from build123d import *

# Parameters (mm, degrees)
BLANKSKE_W         = 300
BLANKSKE_H         = 45
BLANK_DEPTH        = 30
TOOTHCUTSIM_DEPTH  = 305.836021494
TEETHCUTS_COUNT    = 20
TEETHCUTS_PITCH    = 15.70796325
SKETCH1_W          = 305.531648247
SKETCH1_H          = 78.813182986
CUT_EXTRUDE1_DEPTH = 15
SKETCH2_W          = 303.838018684
SKETCH2_H          = 48.852788509
CUT_EXTRUDE2_DEPTH = 26
SKETCH3_W          = 15
SKETCH3_H          = 19
CUT_EXTRUDE3_DEPTH = 138


with BuildPart() as part:
    # BlankSke → Blank (new body)
    with BuildSketch(Plane.XY):
        with Locations((150, 22.5)):
            Rectangle(BLANKSKE_W, BLANKSKE_H)
    extrude(amount=-BLANK_DEPTH)

    # TooCutSkeSim → ToothCutSim (cut, through all)
    with BuildSketch(Plane.XY):
        Polygon((2.153176848, 33.75), (-2.153176848, 33.75), (-6.257086828, 45.0254), (6.257086828, 45.0254), align=None)
    toothcutsim = extrude(amount=-TOOTHCUTSIM_DEPTH, mode=Mode.SUBTRACT)

    # TeethCuts: ToothCutSim ×20
    with Locations(*[(i * TEETHCUTS_PITCH, 0, 0) for i in range(1, TEETHCUTS_COUNT)]):
        add(toothcutsim, mode=Mode.SUBTRACT)

    # Sketch1 → Cut-Extrude1 (cut)
    with BuildSketch(Plane.XY):
        with Locations((152.765824124, 39.406591493)):
            Rectangle(SKETCH1_W, SKETCH1_H)
    extrude(amount=-CUT_EXTRUDE1_DEPTH, mode=Mode.SUBTRACT)

    # Sketch2 → Cut-Extrude2 (cut)
    with BuildSketch(Plane.XZ):
        with Locations((151.919009342, -5.573605746)):
            Rectangle(SKETCH2_W, SKETCH2_H)
    extrude(amount=-CUT_EXTRUDE2_DEPTH, mode=Mode.SUBTRACT)

    # Sketch3 → Cut-Extrude3 (cut)
    with BuildSketch(Plane(origin=(300, 0, 0), x_dir=(0, 0, -1), z_dir=(1, 0, 0))):
        with Locations((22.5, 35.5)):
            Rectangle(SKETCH3_W, SKETCH3_H)
    extrude(amount=-CUT_EXTRUDE3_DEPTH, mode=Mode.SUBTRACT)


solid = part.part
Geometry check sheet. Reference: the model listing, model coordinates, mm. A direction names the side the tool comes from. Coordinates: 2 decimals unless noted, no trailing zeros. Order: outer loops, then holes, each group sorted by start corner. A loop starts at its lowest first (then second) coordinate and runs counter-clockwise, first axis right, second up. Notation, with made-up numbers: (-20, 80.25) - (6, 80.25) arc R28 ccw to (6, 102.25) - close; hole circle Ø1 at (-16, 48.5). An arc over 180 degrees is marked (long way). One line per item, written item: value.
(1) Sectioned sample at C-C (x = 90.5). Enter the section's corners in (y, z).
Data:
outline: (26, -30) - (38.13, -30) - (38.13, -15) - (26, -15) - close
(2) Depth check by flat-ended pin: pin 1 Ø1.1 at (x, z) = (1.5, -19.5) entering from +Y. Enter the tip coordinate at first touch or a pass-through.
Data:
pin 1: stops at y = 33.75
(3) Sectioned sample at B-B (x = 129.5). Enter the section's corners in (y, z).
Data:
outline: (26, -30) - (38.37, -30) - (38.37, -15) - (26, -15) - close
(4) Access from +Z, -Z, +X, -X, +Y, -Y to the whole of each face (thin tool, end or side, straight path). Record for faces 1 (the face through (160.636, 37.605, -22.395)), 2 (the face through (162, 34, -22)).
Data:
face 1: +Z, -Z, +Y
face 2: +Z, -Z, +X, +Y, -Y
(5) Sectioned sample at A-A (y = 38.5). Count the separate pieces of the cut face and the enclosed holes in it, and give its area (3 significant figures).
Data:
separate pieces: 11
enclosed holes: 0
area: 1,210 mm^2
(6) Thickness scan on probe 1 along Y at (x, z) = (96, -24.5). Record the ranges inside material, lowest first. Write a range as from..to.
Data:
probe 1: y = 26..33.75
